The listing builds one solid part. Answer for the finished solid, in the listing's coordinates (mm). A direction names the side the tool comes from. Give positions to 0.01 mm unless a question says otherwise; leave off trailing zeros. Write each loop counter-clockwise with the first axis right and the second up, starting at its lowest first coordinate (ties: lowest second). Pieces come first, ordered by that corner, then holes. Notation, with made-up numbers: (-27.5, 63) -> (16.5, 63) arc R26 cw to (16.5, 99) -> close; hole circle Ø9 at (66, 84.5). An arc over 180 degrees is marked (long way). Use CSV: the item, a comma, the result in double quotes. Start each with the question number.
from build123d import *

# Parameters (mm, degrees)
PAD_DEPTH       = 2.7
SKETCH002_W     = 53
SKETCH002_H     = 6
POCKET_DEPTH    = 1
POCKET001_DEPTH = 2.701
FILLET_R        = 3
CHAMFER_SIZE    = 0.5


with BuildPart() as part:
    # Sketch001 → Pad (new body)
    with BuildSketch(Plane.XY):
        Polygon((-37.25, -23.75), (-37.25, 19.45), (37.25, 19.45), (37.25, -23.75), (43, -23.75), (43, 24.25), (-43, 24.25), (-43, -23.75), align=None)
    extrude(amount=PAD_DEPTH)

    # Sketch002 (on Face9 of Pad) → Pocket (cut)
    with BuildSketch(Plane(origin=(0, 0, 0), x_dir=(1, 0, 0), z_dir=(0, 0, -1))):
        with Locations((0, -21.905725)):
            Rectangle(SKETCH002_W, SKETCH002_H)
    extrude(amount=-POCKET_DEPTH, mode=Mode.SUBTRACT)

    # Sketch003 (on Face4 of Pocket) → Pocket001 (cut, through all)
    with BuildSketch(Plane(origin=(0, 0, 0), x_dir=(1, 0, 0), z_dir=(0, 0, -1))):
        with BuildLine():
            ThreePointArc((38.5, 20), (39.75, 21.25), (38.5, 22.5))
            Line((38.5, 22.5), (36, 22.5))
            Line((36, 22.5), (36, 20))
            Line((38.5, 20), (36, 20))
        make_face()
        with BuildLine():
            ThreePointArc((-38.5, 22.5), (-39.75, 21.25), (-38.5, 20))
            Line((-38.5, 20), (-36, 20))
            Line((-36, 22.5), (-36, 20))
            Line((-38.5, 22.5), (-36, 22.5))
        make_face()
    extrude(amount=-POCKET001_DEPTH, mode=Mode.SUBTRACT)

    # Fillet
    fillet_edges = [part.edges().sort_by_distance(p)[0] for p in [
        (43, -23.75, 1.35),
        (43, 24.25, 1.35),
        (-43, 24.25, 1.35),
        (-43, -23.75, 1.35),
    ]]
    fillet(fillet_edges, radius=FILLET_R)

    # Chamfer
    chamfer_edges = [part.edges().sort_by_distance(p)[0] for p in [
        (-43, 0.25, 0),
        (-42.12132, 23.37132, 0),
        (-42.12132, -22.87132, 0),
        (-33.25, 24.25, 0),
        (-38.625, -23.75, 0),
        (-26.5, 21.85, 0),
        (-37.25, -23.125, 0),
        (-31.875, 19.45, 0),
        (-37.875, -22.5, 0),
        (-37.25, -0.275, 0),
        (-39.75, -21.25, 0),
        (-37.875, -20, 0),
        (33.25, 24.25, 0),
        (42.12132, 23.37132, 0),
        (26.5, 21.85, 0),
        (43, 0.25, 0),
        (31.875, 19.45, 0),
        (42.12132, -22.87132, 0),
        (37.25, -0.275, 0),
        (38.625, -23.75, 0),
        (37.875, -20, 0),
        (37.25, -23.125, 0),
        (39.75, -21.25, 0),
        (37.875, -22.5, 0),
        (-38.625, -23.75, 2.7),
        (-42.12132, -22.87132, 2.7),
        (-37.25, -23.125, 2.7),
        (-43, 0.25, 2.7),
        (-37.875, -22.5, 2.7),
        (-42.12132, 23.37132, 2.7),
        (-39.75, -21.25, 2.7),
        (0, 24.25, 2.7),
        (-37.875, -20, 2.7),
        (42.12132, 23.37132, 2.7),
        (-37.25, -0.275, 2.7),
        (43, 0.25, 2.7),
        (0, 19.45, 2.7),
        (42.12132, -22.87132, 2.7),
        (37.25, -0.275, 2.7),
        (38.625, -23.75, 2.7),
        (37.875, -20, 2.7),
        (37.25, -23.125, 2.7),
        (39.75, -21.25, 2.7),
        (37.875, -22.5, 2.7),
    ]]
    chamfer(chamfer_edges, length=CHAMFER_SIZE)


solid = part.part
Q1. The mould has two halves that part along X. Classify faces 4 (the face through (-6, 21, 2.7)), 5 (the face through (41.843, -22.634, 0.135)), 6 (the face through (37.25, 0, 1)): +X half, -X half, draft (parallel to the pull), parting line (faces both ways), or undercut.
Q2. Straight lines are drawn through the part: L1, parallel to X at y = 17.5, z = 0.7; L2, parallel to Y at x = 36.5, z = 0.7; L3, parallel to X at y = -3, z = 2.3. For each, find the intervals that lie inside material, in ascending order.
Q3. Flat-ended cylindrical pins translate along their axes: pin 1 Ø4 at (x, y) = (3.5, 22.5) entering from -Z; pin 2 Ø8 at (x, y) = (-31.5, 11.5) entering from +Z; pin 3 Ø0.5 at (x, z) = (-1.5, 1.5) entering from -Y; pin 4 Ø1.4 at (y, z) = (-23, 1.5) entering from +X. Find the tip coordinate at first contact, or state that the pin passes through.
Q4. Section B-B on x = 34.5 is taken. Give the vertices of the cut face in (y, z).
Q5. Section A-A on y = 10.5 is taken. Give the vertices of the cut face in (x, z), then the cut area to 4 significant figures.
Q6. For faces 1 (the face through (39.89, -21.28, 0.36)), 2 (the face through (-39.89, -21.28, 2.34)), 3 (the face through (0, 22, 1)), determine the directions among +Z, -Z, +X, -X, +Y, -Y from which every point of the face is accessible in a straight line to the end or side of a thin tool.
Q7. Section C-C on x = 1 is taken. Give the vertices of the cut face in (y, z), then the cut area to 3 significant figures.
Output:
1,face 4,"draft"
1,face 5,"+X half"
1,face 6,"undercut"
2,L1,"-43 to -37.25, 37.25 to 43"
2,L2,"19.45 to 24.25"
2,L3,"-42.9 to -37.35, 37.35 to 42.9"
3,pin 1,"z = 1"
3,pin 2,"through"
3,pin 3,"y = 19.45"
3,pin 4,"x = 42.57"
4,outline,"(19.45, 0.5) -> (19.95, 0) -> (23.75, 0) -> (24.25, 0.5) -> (24.25, 2.2) -> (23.75, 2.7) -> (19.95, 2.7) -> (19.45, 2.2) -> close"
5,outline,"(-43, 0.5) -> (-42.5, 0) -> (-37.75, 0) -> (-37.25, 0.5) -> (-37.25, 2.2) -> (-37.75, 2.7) -> (-42.5, 2.7) -> (-43, 2.2) -> close; (37.25, 0.5) -> (37.75, 0) -> (42.5, 0) -> (43, 0.5) -> (43, 2.2) -> (42.5, 2.7) -> (37.75, 2.7) -> (37.25, 2.2) -> close"
5,area,"30.05 mm²"
6,face 1,"-Z"
6,face 2,"+Z"
6,face 3,"-Z, +Y, -Y"
7,outline,"(19.45, 1) -> (24.25, 1) -> (24.25, 2.2) -> (23.75, 2.7) -> (19.95, 2.7) -> (19.45, 2.2) -> close"
7,area,"7.91 mm²"
